For this review, take the finished solid that the model builds, in its own axes (mm). Face numbers are marked on the shaded views. A direction names the side the tool comes from. Give positions to 0.01 mm unless a question says otherwise; leave off trailing zeros. Loops run counter-clockwise (first coordinate to the right, second up) from the corner with the lowest first, then second, coordinate; pieces in that order, holes last.
```python
from build123d import *

# Parameters (mm, degrees)
SKETCH1_W                    = 27.94
SKETCH1_H                    = 50.8
BASE_FLANGE1_DEPTH           = 0.7366
EDGE_FLANGE1_STRIP_W         = 4.4196
EDGE_FLANGE1_STRIP_H         = 0.7366
EDGE_FLANGE1_STRIP_CUT_DEPTH = 50.8
EDGE_FLANGE1_DEPTH           = 50.8
EDGE_FLANGE1_START           = 0.7366
EDGE_FLANGE1_FLAT_DEPTH      = 0.7366
SKETCH12_R                   = 3.175
CUT_EXTRUDE1_DEPTH           = 53.317865417
CUT_EXTRUDE2_REACH           = 47.698
SKETCH13_R                   = 3.175


# Sheet-metal steps are written as plain solids
with BuildPart() as part:
    # Sketch1 → Base-Flange1 (new body)
    with BuildSketch(Plane(origin=(0, 0, 0), x_dir=(1, 0, 0), z_dir=(0, 1, 0))):
        Rectangle(SKETCH1_W, SKETCH1_H)
    extrude(amount=-BASE_FLANGE1_DEPTH)

    # Edge-Flange1 strip (across the edge) → Edge-Flange1 strip cut (cut)
    with BuildSketch(Plane(origin=(13.97, -0.7366, -25.4), x_dir=(-1, 0, 0), z_dir=(0, 0, 1))):
        with Locations((-1.4732, -0.3683)):
            Rectangle(EDGE_FLANGE1_STRIP_W, EDGE_FLANGE1_STRIP_H)
    edge_flange1_strip_cut = extrude(amount=EDGE_FLANGE1_STRIP_CUT_DEPTH, mode=Mode.SUBTRACT)

    # Edge-Flange1 bend section (across the edge) → Edge-Flange1 (add)
    with BuildSketch(Plane(origin=(13.97, -0.7366, -25.4), x_dir=(-1, 0, 0), z_dir=(0, 0, 1))):
        with BuildLine():
            Line((-0.7366, 0.7366), (0, 0.7366))
            ThreePointArc((0, 0.7366), (0.215745145, 0.215745145), (0.7366, 0))
            Line((0.7366, 0), (0.7366, -0.7366))
            ThreePointArc((0.7366, -0.7366), (-0.30510971, -0.30510971), (-0.7366, 0.7366))
        make_face()
    edge_flange1 = extrude(amount=EDGE_FLANGE1_DEPTH)

    # Edge-Flange1 profile (on flange) → Edge-Flange1 flat (add)
    with BuildSketch(Plane(origin=(13.97, -0.7366, 0), x_dir=(0, 0, 1), z_dir=(1, 0, 0)).offset(EDGE_FLANGE1_START)):
        with BuildLine():
            Line((24.419454366, 7.112682089), (-8.801364085, 32.952298674))
            ThreePointArc((-8.801364085, 32.952298674), (-14.680352055, 33.973299739), (-18.810680555, 29.666870915))
            Line((-18.810680555, 29.666870915), (-25.304272222, 6.688740937))
            ThreePointArc((-25.304272222, 6.688740937), (-25.375954237, 6.346667603), (-25.4, 5.997992571))
            Line((-25.4, 5.997992571), (-25.4, 0.7366))
            Line((-25.4, 0.7366), (25.4, 0.7366))
            Line((25.4, 0.7366), (25.4, 5.10776262))
            ThreePointArc((25.4, 5.10776262), (25.141733342, 6.223689568), (24.419454366, 7.112682089))
        make_face()
    edge_flange1_flat = extrude(amount=-EDGE_FLANGE1_FLAT_DEPTH)

    # Mirror1: Edge-Flange1 strip cut, Edge-Flange1, Edge-Flange1 flat across plane
    add(edge_flange1_strip_cut.mirror(Plane(origin=(0, 0, 0), x_dir=(0, 0, 1), z_dir=(1, 0, 0))), mode=Mode.SUBTRACT)
    add(edge_flange1.mirror(Plane(origin=(0, 0, 0), x_dir=(0, 0, 1), z_dir=(1, 0, 0))))
    add(edge_flange1_flat.mirror(Plane(origin=(0, 0, 0), x_dir=(0, 0, 1), z_dir=(1, 0, 0))))

    # Sketch12 → Cut-Extrude1 (cut, through all)
    with BuildSketch(Plane.ZY.offset(14.7066)):
        with Locations(Location((-12.7, -28.6766, 0), (0, 0, 270))):
            Circle(SKETCH12_R)
    extrude(amount=-CUT_EXTRUDE1_DEPTH, mode=Mode.SUBTRACT)

    # Sketch13 → Cut-Extrude2 (cut, up to next)
    with BuildSketch(Plane(origin=(0, 0, 0), x_dir=(1, 0, 0), z_dir=(0, 1, 0)), mode=Mode.PRIVATE) as cut_extrude2_sk1:
        with Locations(Location((0, 0, 0), (0, 0, 270))):
            Circle(SKETCH13_R)
    cut_extrude2_tool1 = extrude(cut_extrude2_sk1.sketch, amount=-CUT_EXTRUDE2_REACH, mode=Mode.PRIVATE) & part.part
    add(cut_extrude2_tool1.solids().sort_by_distance((0, 0, 0))[0], mode=Mode.SUBTRACT)


solid = part.part
```
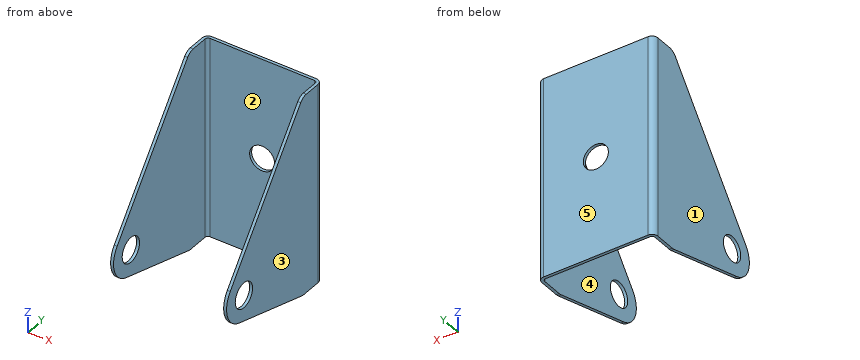
Q1. Consider section C-C on y = -31. Give the boundary of the cut face in (x, z), plus the area to 3 significant figures.
Answers:
outline: (-14.71, -18.61) - (-13.97, -18.61) - (-13.97, -14.86) - (-14.71, -14.86) - close; (-14.71, -10.54) - (-13.97, -10.54) - (-13.97, -5.34) - (-14.71, -5.34) - close; (13.97, -18.61) - (14.71, -18.61) - (14.71, -14.86) - (13.97, -14.86) - close; (13.97, -10.54) - (14.71, -10.54) - (14.71, -5.34) - (13.97, -5.34) - close
area: 13.2 mm2
Q2. Consider section B-B on x = 0. Give the boundary of the cut face in (y, z) (3 decimals).
Answers:
outline: (-0.737, -25.4) - (0, -25.4) - (0, -3.175) - (-0.737, -3.175) - close; (-0.737, 3.175) - (0, 3.175) - (0, 25.4) - (-0.737, 25.4) - close
Q3. Machinability: for the marked faces 4 and 5, which of the approach directions +Z, -Z, +X, -X, +Y, -Y give a long, thin tool a straight path to every point of the face, cutting with its end or side? Answer none if there is none.
Answers:
face 4: +Z, -Z, -Y
face 5: +Z, -Z, +X, -X, +Y
Q4. For probe 1 along X at (y, z) = (-14, 5); probe 2 along Y at (x, z) = (7.5, -17); probe 3 along Y at (x, z) = (-13.5, -14), list the stretches that pass through material, from the lowest coordinate up.
Answers:
probe 1: x = -14.71 to -13.97, 13.97 to 14.71
probe 2: y = -0.74 to 0
probe 3: y = -0.79 to -0.02
Q5. Consider section D-D on y = -17. Give the boundary of the cut face in (x, z).
Answers:
outline: (-14.71, -22.6) - (-13.97, -22.6) - (-13.97, 12.65) - (-14.71, 12.65) - close; (13.97, -22.6) - (14.71, -22.6) - (14.71, 12.65) - (13.97, 12.65) - close
Q6. Mouldability with a two-part tool opening along X and no side actions: class the marked faces 1, 2 and 3 as +X half, -X half, draft (parallel to the pull), parting line (faces both ways), or undercut.
Answers:
face 1: -X half
face 2: undercut
face 3: +X half
Q7. For pin 1 Ø1 at (x, z) = (11.5, 13) entering from -Y; pin 2 Ø2 at (x, z) = (-0.5, -2) entering from -Y; pin 3 Ø10 at (y, z) = (-24.5, 10) entering from -X, all flat-tipped, find the tip position at first contact; note any pin that passes through.
Answers:
pin 1: stops at y = -0.74
pin 2: passes through
pin 3: stops at x = -14.71
Q8. Consider section A-A on z = -12.7. Give the boundary of the cut face in (x, y), plus the area to 3 significant figures.
Answers:
outline: (-14.71, -35.03) - (-13.97, -35.03) - (-13.97, -31.85) - (-14.71, -31.85) - close; (-14.71, -25.5) - (-13.97, -25.5) - (-13.97, -1.47) arc R0.74 cw to (-13.23, -0.74) - (13.23, -0.74) arc R0.74 cw to (13.97, -1.47) - (13.97, -25.5) - (14.71, -25.5) - (14.71, -1.47) arc R1.47 ccw to (13.23, 0) - (-13.23, 0) arc R1.47 ccw to (-14.71, -1.47) - close; (13.97, -35.03) - (14.71, -35.03) - (14.71, -31.85) - (13.97, -31.85) - close
area: 62.1 mm2
